Read the model definition and answer for the solid it produces. Units are mm, in the model's axes. Face numbers are marked on the shaded views. Coordinates: 2 decimals unless noted, no trailing zeros. Order: outer loops, then holes, each group sorted by start corner. A loop starts at its lowest first (then second) coordinate and runs counter-clockwise, first axis right, second up. Notation, with made-up numbers: M -4.5,19.5 L 39.5,19.5 A15 ccw 39.5,43.5 Z; hole C 34.25,-36 d7. An arc over 180 degrees is marked long. Put each result on its own line as item: value.
from build123d import *

# Parameters (mm, degrees)
F0_R     = 10.9855
F1_DEPTH = 25.4


# Not quite as in the source:
# - a feature names something its author has since deleted; it is built from what else it names


with BuildPart() as f1:
    # F0 (on Top) → F1 (new body)
    with BuildSketch(Plane.XY):
        Polygon((53.519200738, -3.5098091407), (27.9298310918, 43.5148113115), (-25.5893696461, 44.8660773572), (-53.519200738, -0.8072770493), (-27.9298310918, -47.8318975015), (25.5893696461, -49.1831635472), align=None)
        with Locations((-30.48, 0)):
            Circle(F0_R, mode=Mode.SUBTRACT)
        with BuildLine():
            ThreePointArc((-10.9855, 0), (0, 10.9855), (10.9855, 0))
            ThreePointArc((10.9855, 0), (0, -10.9855), (-10.9855, 0))
        make_face(mode=Mode.SUBTRACT)
        with BuildLine():
            ThreePointArc((41.4655, 0), (30.48, -10.9855), (19.4945, 0))
            ThreePointArc((19.4945, 0), (30.48, 10.9855), (41.4655, 0))
        make_face(mode=Mode.SUBTRACT)
    extrude(amount=F1_DEPTH)


solid = f1.part
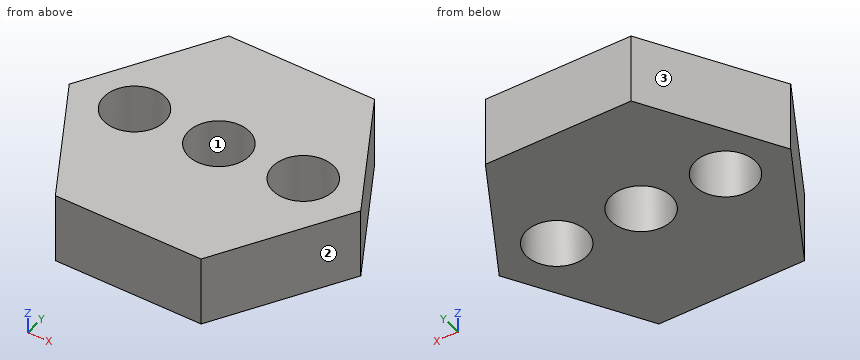
Q1. Find section A-A on x = 0. Write down the section's boundary in (y, z), plus the area to 3 significant figures.
Answers below:
outline: M -48.54,0 L -10.99,0 L -10.99,25.4 L -48.54,25.4 Z; M 10.99,0 L 44.22,0 L 44.22,25.4 L 10.99,25.4 Z
area: 1,800 mm^2
Q2. Consider line 1 along X through (y, z) = (-2.5, 5); line 2 along X through (y, z) = (1, 4.25); line 3 along Y through (x, z) = (-28, 4). Determine where each line is inside the solid, lowest interval first.
Answers below:
line 1: x = -52.6 to -41.18, -19.78 to -10.7, 10.7 to 19.78, 41.18 to 52.97
line 2: x = -52.41 to -41.42, -19.54 to -10.94, 10.94 to 19.54, 41.42 to 51.07
line 3: y = -47.7 to -10.7, 10.7 to 40.92
Q3. For a pull along X with two mould halves and no side action, classify the marked faces 1, 2 and 3 as +X half, -X half, draft (parallel to the pull), parting line (faces both ways), or undercut.
Answers below:
face 1: undercut
face 2: +X half
face 3: -X half
Q4. Find section B-B on z = 15.25. Write down the section's boundary in (x, y).
Answers below:
outline: M -53.52,-0.81 L -27.93,-47.83 L 25.59,-49.18 L 53.52,-3.51 L 27.93,43.51 L -25.59,44.87 Z; hole C -30.48,0 d21.97; hole C 0,0 d21.97; hole C 30.48,0 d21.97
Q5. Given pin 1 (1 mm diameter, centred on x = -10, y = -2, fed in from -Z); pin 2 (1.5 mm diameter, centred on x = -35, z = 4.5, fed in from +Y); pin 3 (2 mm diameter, centred on x = -41.5, z = 8.5, fed in from -Y); pin 4 (1 mm diameter, centred on y = 15.5, z = 14.5, fed in from +X), each flat-ended and moving along its own axis, determine where each tip first touches the part or whether it passes through.
Answers below:
pin 1: passes through
pin 2: stops at y = 30.7
pin 3: stops at y = -24.73
pin 4: stops at x = 43.45
Q6. Find section C-C on y = 9. Write down the section's boundary in (x, z).
Answers below:
outline: M -47.52,0 L -36.78,0 L -36.78,25.4 L -47.52,25.4 Z; M -24.18,0 L -6.3,0 L -6.3,25.4 L -24.18,25.4 Z; M 6.3,0 L 24.18,0 L 24.18,25.4 L 6.3,25.4 Z; M 36.78,0 L 46.71,0 L 46.71,25.4 L 36.78,25.4 Z
Q7. Find section D-D on x = 30.48. Write down the section's boundary in (y, z).
Answers below:
outline: M -41.19,0 L -10.99,0 L -10.99,25.4 L -41.19,25.4 Z; M 10.99,0 L 38.83,0 L 38.83,25.4 L 10.99,25.4 Z
